For this review, take the finished solid that the model builds, in its own axes (mm). Give positions to 0.01 mm unless a question says otherwise; leave off trailing zeros. Loops run counter-clockwise (first coordinate to the right, second up) from the corner with the lowest first, then second, coordinate; pieces in that order, holes last. Notation, with made-up numbers: (-31.5, 11.25) - (27.5, 11.25) arc R27 ccw to (27.5, 47.25) - close; hole circle Ø1 at (51, -7.75). An arc over 180 degrees is marked (long way). Put each result on its own line as item: value.
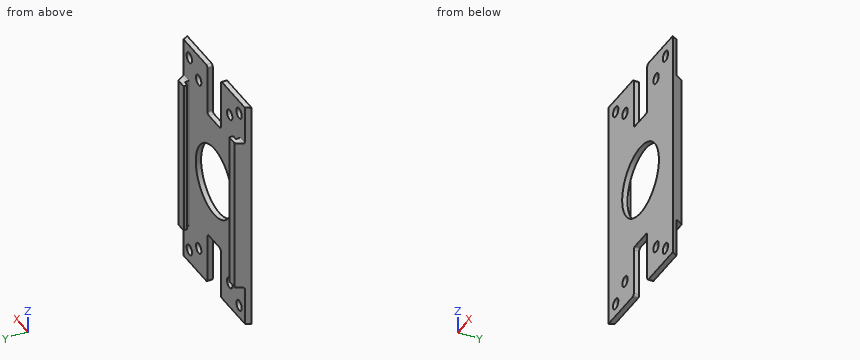
from build123d import *

# Parameters (mm, degrees)
BOSS_EXTRUDE1_DEPTH     = 180
SKETCH2_W               = 91.64
SKETCH2_H               = 8.017032047
CUT_EXTRUDE1_DEPTH      = 30
SKETCH3_W               = 91.64
SKETCH3_H               = 8.483725915
CUT_EXTRUDE2_DEPTH      = 30
FILLET1_R               = 1
FILLET2_R               = 1
FILLET3_R               = 1
CUT_EXTRUDE3_DEPTH      = 200.729129072
CUT_EXTRUDE3_DEPTH_BACK = 200.729129072
SKETCH4_R               = 4
SKETCH4_R_2             = 27.5


with BuildPart() as part:
    # Sketch1 → Boss-Extrude1 (new body)
    with BuildSketch(Plane.XY):
        with BuildLine():
            Line((-80.35, -4.05), (-79.85, -4.05))
            Line((-79.85, -4.05), (3.65, -4.05))
            Line((3.65, -4.05), (4.15, -4.05))
            Line((4.15, -4.05), (10.15, -4.05))
            Line((10.15, -4.05), (4.295651273, 5.707247878))
            ThreePointArc((4.295651273, 5.707247878), (4.113254218, 5.885099953), (3.866904811, 5.95))
            Line((3.866904811, 5.95), (3.65, 5.95))
            Line((3.65, 5.95), (-3.35, 5.95))
            ThreePointArc((-3.35, 5.95), (-3.703553391, 5.803553391), (-3.85, 5.45))
            Line((-3.85, 5.45), (-3.85, 3.45))
            ThreePointArc((-3.85, 3.45), (-3.703553391, 3.096446609), (-3.35, 2.95))
            Line((-3.35, 2.95), (-0.35, 2.95))
            ThreePointArc((-0.35, 2.95), (0.003553391, 2.803553391), (0.15, 2.45))
            Line((0.15, 2.45), (0.15, 0.5))
            ThreePointArc((0.15, 0.5), (0.003553391, 0.146446609), (-0.35, 0))
            Line((-0.35, 0), (-75.85, 0))
            ThreePointArc((-75.85, 0), (-76.203553391, 0.146446609), (-76.35, 0.5))
            Line((-76.35, 0.5), (-76.35, 2.45))
            ThreePointArc((-76.35, 2.45), (-76.203553391, 2.803553391), (-75.85, 2.95))
            Line((-75.85, 2.95), (-72.85, 2.95))
            ThreePointArc((-72.85, 2.95), (-72.496446609, 3.096446609), (-72.35, 3.45))
            Line((-72.35, 3.45), (-72.35, 5.45))
            ThreePointArc((-72.35, 5.45), (-72.496446609, 5.803553391), (-72.85, 5.95))
            Line((-72.85, 5.95), (-79.85, 5.95))
            Line((-79.85, 5.95), (-80.066904811, 5.95))
            ThreePointArc((-80.066904811, 5.95), (-80.313254218, 5.885099953), (-80.495651273, 5.707247878))
            Line((-80.495651273, 5.707247878), (-86.35, -4.05))
            Line((-86.35, -4.05), (-80.35, -4.05))
        make_face()
    extrude(amount=BOSS_EXTRUDE1_DEPTH)

    # Sketch2 → Cut-Extrude1 (cut)
    with BuildSketch(Plane.XY.offset(180)):
        with Locations((-38.1, 4.008516024)):
            Rectangle(SKETCH2_W, SKETCH2_H)
    extrude(amount=-CUT_EXTRUDE1_DEPTH, mode=Mode.SUBTRACT)

    # Sketch3 → Cut-Extrude2 (cut)
    with BuildSketch(Plane(origin=(0, 0, 0), x_dir=(-1, 0, 0), z_dir=(0, 0, -1))):
        with Locations((38.1, 4.241862958)):
            Rectangle(SKETCH3_W, SKETCH3_H)
    extrude(amount=-CUT_EXTRUDE2_DEPTH, mode=Mode.SUBTRACT)

    # Fillet1
    fillet1_edges = [part.edges().sort_by_distance(p)[0] for p in [
        (-79.885, 0, 150),
    ]]
    fillet(fillet1_edges, radius=FILLET1_R)

    # Fillet2
    fillet2_edges = [part.edges().sort_by_distance(p)[0] for p in [
        (3.685, 0, 150),
    ]]
    fillet(fillet2_edges, radius=FILLET2_R)

    # Fillet3
    fillet3_edges = [part.edges().sort_by_distance(p)[0] for p in [
        (-79.885, 0, 30),
        (3.685, 0, 30),
    ]]
    fillet(fillet3_edges, radius=FILLET3_R)

    # Sketch4 → Cut-Extrude3 (cut, two sides: drawn at the far end of the back side and taken through both)
    with BuildSketch(Plane(origin=(0, 0, 0), x_dir=(1, 0, 0), z_dir=(0, 1, 0)).offset(-CUT_EXTRUDE3_DEPTH_BACK)):
        with BuildLine():
            Line((-28.1, -38), (-28.1, -2))
            ThreePointArc((-28.1, -2), (-27.514213562, -0.585786438), (-26.1, 0))
            Line((-26.1, 0), (-50.1, 0))
            ThreePointArc((-50.1, 0), (-48.685786438, -0.585786438), (-48.1, -2))
            Line((-48.1, -2), (-48.1, -38))
            ThreePointArc((-48.1, -38), (-47.514213562, -39.414213562), (-46.1, -40))
            Line((-46.1, -40), (-30.1, -40))
            ThreePointArc((-30.1, -40), (-28.685786438, -39.414213562), (-28.1, -38))
        make_face()
        with Locations(Location((-75.35, -10, 0), (0, 0, 270))):
            Circle(SKETCH4_R)
        with Locations(Location((-61.35, -20, 0), (0, 0, 270))):
            Circle(SKETCH4_R)
        with Locations(Location((-14.85, -20, 0), (0, 0, 270))):
            Circle(SKETCH4_R)
        with Locations(Location((-0.85, -10, 0), (0, 0, 270))):
            Circle(SKETCH4_R)
        with Locations(Location((-38.1, -90, 0), (0, 0, 270))):
            Circle(SKETCH4_R_2)
        with BuildLine():
            ThreePointArc((-30.1, -140), (-28.685786438, -140.585786438), (-28.1, -142))
            Line((-28.1, -142), (-28.1, -178))
            ThreePointArc((-28.1, -178), (-27.514213562, -179.414213562), (-26.1, -180))
            Line((-26.1, -180), (-50.1, -180))
            ThreePointArc((-50.1, -180), (-48.685786438, -179.414213562), (-48.1, -178))
            Line((-48.1, -178), (-48.1, -142))
            ThreePointArc((-48.1, -142), (-47.514213562, -140.585786438), (-46.1, -140))
            Line((-46.1, -140), (-30.1, -140))
        make_face()
        with Locations(Location((-61.35, -160, 0), (0, 0, 270))):
            Circle(SKETCH4_R)
        with Locations(Location((-75.35, -170, 0), (0, 0, 270))):
            Circle(SKETCH4_R)
        with Locations(Location((-14.85, -160, 0), (0, 0, 270))):
            Circle(SKETCH4_R)
        with Locations(Location((-0.85, -170, 0), (0, 0, 270))):
            Circle(SKETCH4_R)
    extrude(amount=CUT_EXTRUDE3_DEPTH + CUT_EXTRUDE3_DEPTH_BACK, mode=Mode.SUBTRACT)


solid = part.part
1) Take a section at D-D on x = -14.85. State the section outline as (y, z) points, and give its area (3 significant figures).
Geometry check:
outline: (-4.05, 0) - (0, 0) - (0, 16) - (-4.05, 16) - close; (-4.05, 24) - (0, 24) - (0, 75.31) - (-4.05, 75.31) - close; (-4.05, 104.69) - (0, 104.69) - (0, 156) - (-4.05, 156) - close; (-4.05, 164) - (0, 164) - (0, 180) - (-4.05, 180) - close
area: 545 mm²
2) Take a section at A-A on x = -38.1. State the section outline as (y, z) points.
Geometry check:
outline: (-4.05, 40) - (0, 40) - (0, 62.5) - (-4.05, 62.5) - close; (-4.05, 117.5) - (0, 117.5) - (0, 140) - (-4.05, 140) - close
3) Wall thickness on line 1 (Z direction, x = -0.85, y = -2.3); line 2 (X direction, y = -2.85, z = 10); line 3 (X direction, y = -0.8, z = 10): over which ranges is each line inside the solid? List them lowest first.
Geometry check:
line 1: z = 0 to 6, 14 to 166, 174 to 180
line 2: x = -85.63 to -79.35, -71.35 to -48.1, -28.1 to -4.85, 3.15 to 9.43
line 3: x = -84.4 to -79.35, -71.35 to -48.1, -28.1 to -4.85, 3.15 to 8.2
4) Take a section at B-B on z = 170. State the section outline as (x, y) points.
Geometry check:
outline: (-86.35, -4.05) - (-79.35, -4.05) - (-79.35, 0) - (-83.92, 0) - close; (-71.35, -4.05) - (-48.1, -4.05) - (-48.1, 0) - (-71.35, 0) - close; (-28.1, -4.05) - (-4.85, -4.05) - (-4.85, 0) - (-28.1, 0) - close; (3.15, -4.05) - (10.15, -4.05) - (7.72, 0) - (3.15, 0) - close
5) Insertion check: pin 1 Ø10.5 at (x, z) = (-75.35, 10) entering from +Y; pin 2 Ø1.5 at (x, y) = (1.5, 4) entering from +Z; pin 3 Ø1.5 at (x, y) = (-76, 4) entering from -Z; pin 4 Ø7 at (x, z) = (-61.35, 20) entering from -Y. Each pin has a flat end and moves straight along its axis. Give the tip position at first contact, or say it passes through.
Geometry check:
pin 1: stops at y = 0
pin 2: stops at z = 150
pin 3: stops at z = 30
pin 4: passes through
6) Take a section at C-C on z = 102. State the section outline as (x, y) points, and give its area (3 significant figures).
Geometry check:
outline: (-86.35, -4.05) - (-62.84, -4.05) - (-62.84, 0) - (-75.85, 0) arc R0.5 cw to (-76.35, 0.5) - (-76.35, 2.45) arc R0.5 cw to (-75.85, 2.95) - (-72.85, 2.95) arc R0.5 ccw to (-72.35, 3.45) - (-72.35, 5.45) arc R0.5 ccw to (-72.85, 5.95) - (-80.07, 5.95) arc R0.5 ccw to (-80.5, 5.71) - close; (-13.36, -4.05) - (10.15, -4.05) - (4.3, 5.71) arc R0.5 ccw to (3.87, 5.95) - (-3.35, 5.95) arc R0.5 ccw to (-3.85, 5.45) - (-3.85, 3.45) arc R0.5 ccw to (-3.35, 2.95) - (-0.35, 2.95) arc R0.5 cw to (0.15, 2.45) - (0.15, 0.5) arc R0.5 cw to (-0.35, 0) - (-13.36, 0) - close
area: 273 mm²
